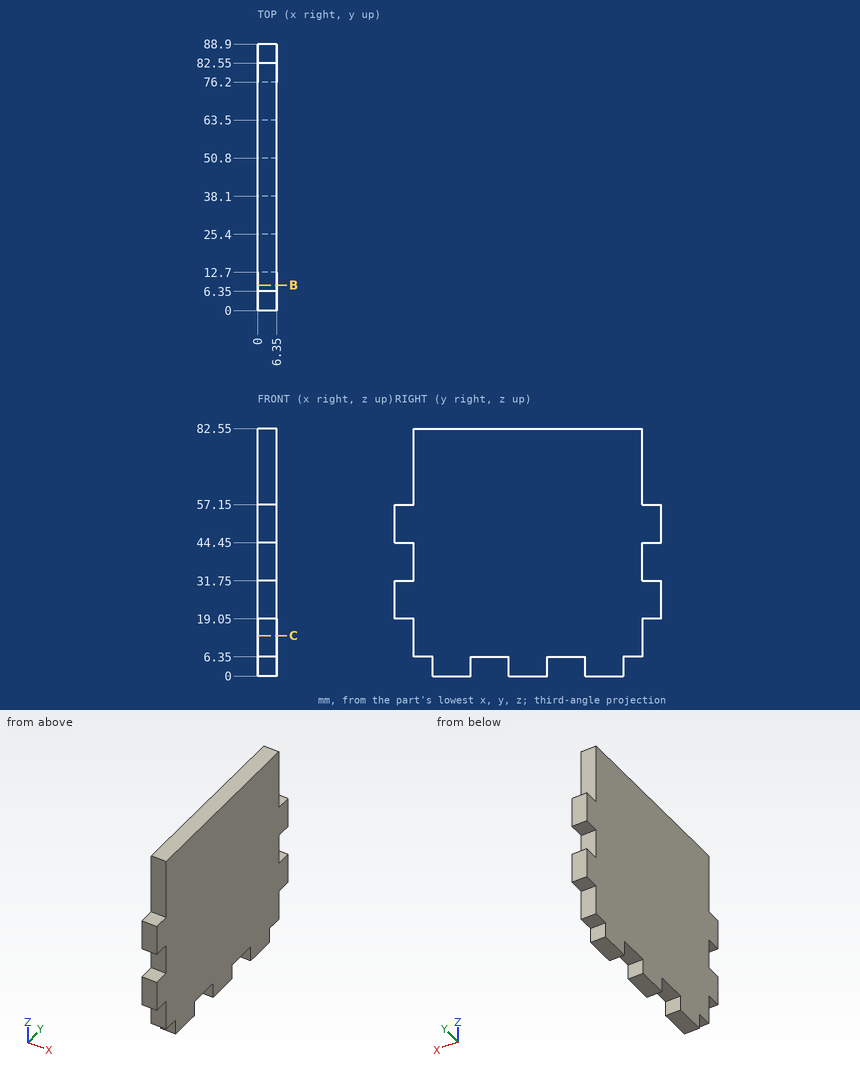
Could you check a few things on this drawing? It's one solid part, dimensions in mm from its lowest x, y, z. Give positions to 0.01 mm unless a question says otherwise; leave off trailing zeros. Write each loop counter-clockwise with the first axis right and the second up, starting at its lowest first coordinate (ties: lowest second). Pieces come first, ordered by that corner, then holes. Notation, with made-up numbers: (15.5, -37) - (65.5, -37) arc R29 cw to (65.5, -6) - close; hole circle Ø10 at (84.5, 3). An arc over 180 degrees is marked (long way). Use CSV: the item, a comma, the result in double quotes. Start each with the question number.
Item 1: I want a section at B-B, the plane y = 8.5. Please give me the cut outline in (x, z).
Item 2: I'm going to push flat-ended pins straight in: pin 1 (3 mm diameter, centred on x = 2.5, y = 85, fed in from +Z); pin 2 (1.9 mm diameter, centred on x = 3, y = 8, fed in from -Z); pin 3 (3 mm diameter, centred on x = 4, z = 14, fed in from -Y). Where does each tip first touch, or does it pass through?
Item 3: If I drill on line 1 along Y through (x, z) = (2.5, 4); line 2 along Y through (x, z) = (5, 71), over which ranges is the centre line in solid material (lowest first)?
Findings:
1,outline,"(0, 6.35) - (6.35, 6.35) - (6.35, 82.55) - (0, 82.55) - close"
2,pin 1,"stops at z = 57.15"
2,pin 2,"stops at z = 6.35"
2,pin 3,"stops at y = 6.35"
3,line 1,"y = 12.7 to 25.4, 38.1 to 50.8, 63.5 to 76.2"
3,line 2,"y = 6.35 to 82.55"
